```python
from build123d import *

# Parameters (mm, degrees)
ESBO_O3_W                = 400
ESBO_O3_H                = 154
RESSALTO_EXTRUS_O1_DEPTH = 1.5
ESBO_O10_W               = 60
ESBO_O10_H               = 39
ESBO_O10_W_2             = 100
CORTE_EXTRUS_O1_DEPTH    = 429.623669435
ESBO_O11_R               = 10
ESBO_O11_R_2             = 2.5
CORTE_EXTRUS_O2_DEPTH    = 429.623669435
DOBRA_START              = -400
DOBRA_ESBO_ADA1_DEPTH    = 400
DOBRA_ESBO_ADA1_2_DEPTH  = 100
DOBRA_START_2            = -60
DOBRA_ESBO_ADA1_3_DEPTH  = 60
DOBRA_START_3            = -300
DOBRA_ESBO_ADA1_4_DEPTH  = 240
DOBRA_ESBO_ADA1_5_DEPTH  = 400
DOBRA_ESBO_ADA2_DEPTH    = 400
DOBRA_ESBO_ADA2_2_DEPTH  = 100
DOBRA_ESBO_ADA2_3_DEPTH  = 60
DOBRA_ESBO_ADA2_4_DEPTH  = 240
DOBRA_ESBO_ADA2_5_DEPTH  = 400


# Read off the part's stored shape, not the designer's step: Transforma__o de esbo_o2, Dobra esbo_ada2
with BuildPart() as part:
    # Esboço3 → Ressalto-extrusão1 (new body)
    with BuildSketch(Plane(origin=(0, 0, 0), x_dir=(0, 0, -1), z_dir=(1, 0, 0))):
        with Locations((200, 77)):
            Rectangle(ESBO_O3_W, ESBO_O3_H)
    extrude(amount=RESSALTO_EXTRUS_O1_DEPTH)

    # Esboço10 → Corte-extrusão1 (cut, through all)
    with BuildSketch(Plane.ZY):
        with Locations((-30, 134.5)):
            Rectangle(ESBO_O10_W, ESBO_O10_H)
        with Locations((-350, 134.5)):
            Rectangle(ESBO_O10_W_2, ESBO_O10_H)
        with Locations((-350, 19.5)):
            Rectangle(ESBO_O10_W_2, ESBO_O10_H)
        with Locations((-30, 19.5)):
            Rectangle(ESBO_O10_W, ESBO_O10_H)
    extrude(amount=-CORTE_EXTRUS_O1_DEPTH, mode=Mode.SUBTRACT)

    # Esboço11 → Corte-extrusão2 (cut, through all)
    with BuildSketch(Plane(origin=(1.5, 0, 0), x_dir=(0, 0, -1), z_dir=(1, 0, 0))):
        with Locations((30, 57)):
            Circle(ESBO_O11_R)
        with Locations(Location((30, 97, 0), (0, 0, 180))):
            Circle(ESBO_O11_R)
        with Locations((11.75, 57)):
            Circle(ESBO_O11_R_2)
        with Locations((48.25, 57)):
            Circle(ESBO_O11_R_2)
        with Locations(Location((48.25, 97, 0), (0, 0, 180))):
            Circle(ESBO_O11_R_2)
        with Locations(Location((11.75, 97, 0), (0, 0, 180))):
            Circle(ESBO_O11_R_2)
    extrude(amount=-CORTE_EXTRUS_O2_DEPTH, mode=Mode.SUBTRACT)

    # Dobra esboçada1 outline → Dobra esboçada1 (cut)
    with BuildSketch(Plane.XY.offset(DOBRA_START)):
        with BuildLine():
            Line((1.5, 0), (1.5, 38.287563626))
            ThreePointArc((1.5, 38.287563626), (0.397581589, 39.539659775), (0, 41.159844949))
            Line((0, 41.159844949), (0, 0))
            Line((0, 0), (1.5, 0))
        make_face()
    extrude(amount=DOBRA_ESBO_ADA1_DEPTH, mode=Mode.SUBTRACT)

    # Dobra esbo_ada1 2 outline → Dobra esbo_ada1 2 (cut)
    with BuildSketch(Plane.XY.offset(DOBRA_START)):
        Polygon((1.5, 39), (1.5, 39.159844949), (1.340155051, 39), align=None)
    extrude(amount=DOBRA_ESBO_ADA1_2_DEPTH, mode=Mode.SUBTRACT)

    # Dobra esbo_ada1 3 outline → Dobra esbo_ada1 3 (cut)
    with BuildSketch(Plane.XY.offset(DOBRA_START_2)):
        Polygon((1.5, 39), (1.5, 39.159844949), (1.340155051, 39), align=None)
    extrude(amount=DOBRA_ESBO_ADA1_3_DEPTH, mode=Mode.SUBTRACT)

    # Dobra esbo_ada1 4 outline → Dobra esbo_ada1 4 (add)
    with BuildSketch(Plane.XY.offset(DOBRA_START_3)):
        with BuildLine():
            Line((40.340155051, 39.159844949), (3.5, 39.159844949))
            ThreePointArc((3.5, 39.159844949), (2.085786438, 39.745631387), (1.5, 41.159844949))
            Line((1.5, 41.159844949), (1.5, 38.287563626))
            ThreePointArc((1.5, 38.287563626), (2.451902827, 37.820459929), (3.5, 37.659844949))
            Line((3.5, 37.659844949), (40.340155051, 37.659844949))
            Line((40.340155051, 37.659844949), (40.340155051, 39.159844949))
        make_face()
    extrude(amount=DOBRA_ESBO_ADA1_4_DEPTH)

    # Dobra esbo_ada1 5 outline → Dobra esbo_ada1 5 (add)
    with BuildSketch(Plane.XY.offset(DOBRA_START)):
        with BuildLine():
            Line((1.5, 39.159844949), (2.085786438, 39.745631387))
            ThreePointArc((2.085786438, 39.745631387), (1.652240935, 40.394478084), (1.5, 41.159844949))
            Line((1.5, 41.159844949), (1.5, 39.159844949))
        make_face()
        with BuildLine():
            Line((1.025126266, 38.684971215), (1.340155051, 39))
            Line((1.340155051, 39), (0.745899458, 39))
            ThreePointArc((0.745899458, 39), (0.880772294, 38.838283789), (1.025126266, 38.684971215))
        make_face()
    extrude(amount=DOBRA_ESBO_ADA1_5_DEPTH)

    # Dobra esboçada2 outline → Dobra esboçada2 (cut)
    with BuildSketch(Plane.XY.offset(DOBRA_START)):
        with BuildLine():
            Line((1.5, 115.712436374), (1.5, 154))
            Line((1.5, 154), (0, 154))
            Line((0, 154), (0, 112.840155051))
            ThreePointArc((0, 112.840155051), (0.397581589, 114.460340225), (1.5, 115.712436374))
        make_face()
    extrude(amount=DOBRA_ESBO_ADA2_DEPTH, mode=Mode.SUBTRACT)

    # Dobra esbo_ada2 2 outline → Dobra esbo_ada2 2 (cut)
    with BuildSketch(Plane.XY.offset(DOBRA_START)):
        Polygon((1.5, 114.840155051), (1.5, 115), (1.340155051, 115), align=None)
    extrude(amount=DOBRA_ESBO_ADA2_2_DEPTH, mode=Mode.SUBTRACT)

    # Dobra esbo_ada2 3 outline → Dobra esbo_ada2 3 (cut)
    with BuildSketch(Plane.XY.offset(DOBRA_START_2)):
        Polygon((1.5, 114.840155051), (1.5, 115), (1.340155051, 115), align=None)
    extrude(amount=DOBRA_ESBO_ADA2_3_DEPTH, mode=Mode.SUBTRACT)

    # Dobra esbo_ada2 4 outline → Dobra esbo_ada2 4 (add)
    with BuildSketch(Plane.XY.offset(DOBRA_START_3)):
        with BuildLine():
            Line((40.340155051, 114.840155051), (40.340155051, 116.340155051))
            Line((40.340155051, 116.340155051), (3.5, 116.340155051))
            ThreePointArc((3.5, 116.340155051), (2.451902827, 116.179540071), (1.5, 115.712436374))
            Line((1.5, 115.712436374), (1.5, 112.840155051))
            ThreePointArc((1.5, 112.840155051), (2.085786438, 114.254368613), (3.5, 114.840155051))
            Line((3.5, 114.840155051), (40.340155051, 114.840155051))
        make_face()
    extrude(amount=DOBRA_ESBO_ADA2_4_DEPTH)

    # Dobra esbo_ada2 5 outline → Dobra esbo_ada2 5 (add)
    with BuildSketch(Plane.XY.offset(DOBRA_START)):
        with BuildLine():
            ThreePointArc((1.5, 112.840155051), (1.652240935, 113.605521916), (2.085786438, 114.254368613))
            Line((2.085786438, 114.254368613), (1.5, 114.840155051))
            Line((1.5, 114.840155051), (1.5, 112.840155051))
        make_face()
        with BuildLine():
            Line((1.340155051, 115), (1.025126266, 115.315028785))
            ThreePointArc((1.025126266, 115.315028785), (0.880772294, 115.161716211), (0.745899458, 115))
            Line((0.745899458, 115), (1.340155051, 115))
        make_face()
    extrude(amount=DOBRA_ESBO_ADA2_5_DEPTH)


solid = part.part
```
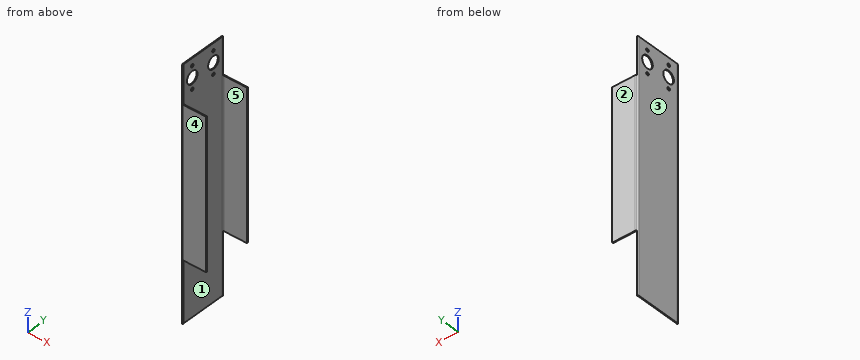
CAD build for the part. Positions are in the model's coordinates, mm. Face numbers are marked on the shaded views. A direction names the side the tool comes from. Round coordinates to 2 decimals unless told otherwise and drop trailing zeros. Order: outer loops, then holes, each group sorted by start corner. A loop starts at its lowest first (then second) coordinate and runs counter-clockwise, first axis right, second up.
Q1. Wall check: L1, parallel to Z at x = 0.95, y = 97; L2, parallel to Y at x = 14, z = -99.5; L3, parallel to Y at x = 0.4, z = -48.25. Give the ranges that are in metal, low to high.
Q2. Which spindle directions (+Z, -Z, +X, -X, +Y, -Y) get a long thin tool onto all of the face, cutting with end or side? Do the marked faces 1 and 2. Say none if no direction does.
Q3. Slice it at C-C (z = -73). Write the cut outline in (x, y).
Q4. Slice it at D-D (y = 76.5). Write the cut outline in (x, z).
Q5. Drop flat-ended pins along their axis: pin 1 (1 mm diameter, centred on x = 25.5, y = 39, fed in from +Z); pin 2 (8 mm diameter, centred on y = 57, z = -48.25, fed in from +X); pin 3 (2.5 mm diameter, centred on x = 16.5, y = 38.5, fed in from -Z); pin 4 (12 mm diameter, centred on x = 25.5, y = 104.5, fed in from -Z). Give the stop position or say it passes through.
Q6. Slice it at B-B (x = 34). Write the cut outline in (y, z), and give its area (3 significant figures).
Q7. Slice it at A-A (z = -30). Write the cut outline in (x, y), and give its area (3 significant figures).
Q8. Two-plate mould, pull along Y, no slides. Class the marked faces 3, 4 and 5: pulls with the +Y half, pulls with the -Y half, needs draft (parallel to the pull), parting line crosses it, or undercut.
Results below:
1. L1: z = -400 to -50.75, -45.75 to -40, -20 to -14.25, -9.25 to 0
1. L2: y = 37.66 to 39.16, 114.84 to 116.34
1. L3: y = 39.54 to 54.5, 59.5 to 94.5, 99.5 to 114.46
2. face 1: +Z, -Z, +X
2. face 2: +Z, -Z, +X, -X, +Y
3. outline: (0, 41.16) arc R3.5 ccw to (3.5, 37.66) - (40.34, 37.66) - (40.34, 39.16) - (3.5, 39.16) arc R2 cw to (1.5, 41.16) - (1.5, 112.84) arc R2 cw to (3.5, 114.84) - (40.34, 114.84) - (40.34, 116.34) - (3.5, 116.34) arc R3.5 ccw to (0, 112.84) - close
4. outline: (0, -400) - (1.5, -400) - (1.5, 0) - (0, 0) - close
5. pin 1: stops at z = -60
5. pin 2: stops at x = 1.5
5. pin 3: stops at z = -300
5. pin 4: passes through
6. outline: (37.66, -300) - (39.16, -300) - (39.16, -60) - (37.66, -60) - close; (114.84, -300) - (116.34, -300) - (116.34, -60) - (114.84, -60) - close
6. area: 720 mm2
7. outline: (0, 41.16) arc R3.5 ccw to (1.03, 38.68) - (2.09, 39.75) arc R2 cw to (1.5, 41.16) - (1.5, 47) - (0, 47) - close; (0, 67) - (1.5, 67) - (1.5, 87) - (0, 87) - close; (0, 107) - (1.5, 107) - (1.5, 112.84) arc R2 cw to (2.09, 114.25) - (1.03, 115.32) arc R3.5 ccw to (0, 112.84) - close
7. area: 54.0 mm2
8. face 3: needs draft
8. face 4: pulls with the -Y half
8. face 5: undercut
